from build123d import *

# Parameters (mm, degrees)
F1_DEPTH = 7.5
F2_SIZE  = 7.49999


# Not quite as in the source:
# - a fillet or chamfer is up to 0.001 mm smaller than in the source, because OpenCascade refuses the exact size


with BuildPart() as f1:
    # F0 (on Front) → F1 (new body)
    with BuildSketch(Plane.XZ):
        with BuildLine():
            Line((-86.7414106019, 13.5850626232), (-86.7414106019, -6.4149373768))
            ThreePointArc((-86.7414106019, -6.4149373768), (-49.5427734858, 0.7956791903), (-11.7279719579, 3.1982569702))
            Line((-11.7279719579, 3.1982569702), (-11.7279719579, 23.1982569702))
            ThreePointArc((-11.7279719579, 23.1982569702), (-49.5427734858, 20.7956791903), (-86.7414106019, 13.5850626232))
        make_face()
    extrude(amount=F1_DEPTH)

    # F2 (size 7.5 in the source; OpenCascade refuses exactly that, so slightly less here)
    f2_edges = [f1.edges().sort_by_distance(p)[0] for p in [
        (-11.727972, -7.5, 13.198257),
    ]]
    chamfer(f2_edges, length=F2_SIZE)


solid = f1.part
The listing builds one solid part. Answer for the finished solid, in the listing's coordinates (mm). Round coordinates to 2 decimals unless told otherwise and drop trailing zeros. Write each loop counter-clockwise with the first axis right and the second up, starting at its lowest first coordinate (ties: lowest second). Pieces come first, ordered by that corner, then holes. Notation, with made-up numbers: (53.25, -22.75) - (96.25, -22.75) arc R8 ccw to (96.25, -13.75) - close; hole circle Ø5 at (44, 44). An arc over 180 degrees is marked (long way). Use a Markdown table: item, result. Add a question column.
1. Flat-ended cylindrical pins translate along their axes: P1, Ø12, axis at x = -41.5, z = 1.5, coming from the +Y side; P2, Ø4, axis at x = -76.5, y = -5, coming from the +Z side; P3, Ø1.5, axis at x = -52, y = -1.5, coming from the -Z side; P4, Ø4, axis at x = -49, y = -2.5, coming from the +Z side. Find the tip coordinate at first contact, or state that the pin passes through.
2. The part is cut by section C-C (x = -22.5). Write down the section's boundary in (y, z).
3. The part is cut by section B-B (y = -2.25). Write down the section's boundary in (x, z), and give its area (3 significant figures).
4. Consider line 1 (Z direction, x = -19.5, y = -0.75); line 2 (X direction, y = -3.75, z = 10); line 3 (Z direction, x = -61.5, y = -1.5). Determine where each line is inside the solid, lowest interval first.
Reported:
| question | item | result |
|---|---|---|
| 1 | P1 | y = 0 |
| 1 | P2 | z = 16.51 |
| 1 | P3 | z = 0.37 |
| 1 | P4 | z = 21.11 |
| 2 | outline | (-7.5, 3.01) - (0, 3.01) - (0, 23.01) - (-7.5, 23.01) - close |
| 3 | outline | (-86.74, -6.41) arc R296.19 cw to (-13.98, 3.19) - (-13.98, 23.19) arc R296.19 ccw to (-86.74, 13.59) - close |
| 3 | area | 1,460 mm^2 |
| 4 | line 1 | 3.1 to 23.1 |
| 4 | line 2 | -86.74 to -15.48 |
| 4 | line 3 | -0.99 to 19.01 |
